```python
from build123d import *

# Parameters (mm, degrees)
F_1_4_20_TAPPED_HOLE1_D = 5.1054
SKETCH4_W               = 4.064
SKETCH4_H               = 3.0734
CHAMFER1_SIZE           = 0.127
F_8_32_TAPPED_HOLE1_D   = 3.4544
CUT_EXTRUDE1_REACH      = 182.054
SKETCH7_W               = 50.8
SKETCH7_H               = 2.565921067


with BuildPart() as part:
    # Sketch1 → Revolve1 (revolve)
    with BuildSketch(Plane.XY, mode=Mode.PRIVATE) as revolve1_sk:
        Polygon((109.7915, 0), (109.7915, 2.54), (105.7783, 2.54), (80.3783, 2.54), (80.3783, 12.7), (105.7783, 12.7), (127, 12.7), (127, 0), align=None)
    revolve(revolve1_sk.sketch.rotate(Axis((0, 0, 0), (0, 1, 0)), 90), axis=Axis((0, 0, 0), (0, 1, 0)))

    # 1/4-20 Tapped Hole1 (through all)
    with Locations(Plane(origin=(0, 12.7, 0), x_dir=(1, 0, 0), z_dir=(0, 1, 0))):
        with Locations((0, 118.745), (59.3725, 102.836186572), (102.836186572, 59.3725), (118.745, 0), (102.836186572, -59.3725), (59.3725, -102.836186572), (0, -118.745), (-59.3725, -102.836186572), (-102.836186572, -59.3725), (-118.745, 0), (-102.836186572, 59.3725), (-59.3725, 102.836186572)):
            Hole(F_1_4_20_TAPPED_HOLE1_D / 2)

    # Sketch4 → Cut-Revolve1 (revolve, cut)
    with BuildSketch(Plane.XY, mode=Mode.PRIVATE) as cut_revolve1_sk:
        with Locations((109.7788, 11.1633)):
            Rectangle(SKETCH4_W, SKETCH4_H)
    revolve(cut_revolve1_sk.sketch.rotate(Axis((0, 12.7, 0), (0, -1, 0)), 90), axis=Axis((0, 12.7, 0), (0, -1, 0)), mode=Mode.SUBTRACT)

    # Chamfer1
    chamfer1_edges = [part.edges().sort_by_distance(p)[0] for p in [
        (0, 12.7, -107.7468),
        (0, 12.7, -111.8108),
    ]]
    chamfer(chamfer1_edges, length=CHAMFER1_SIZE)

    # #8-32 Tapped Hole1 (through all)
    with Locations(Plane(origin=(0, 2.54, 0), x_dir=(-1, 0, 0), z_dir=(0, -1, 0))):
        with Locations((6.35, -85.09), (-6.35, -85.09)):
            Hole(F_8_32_TAPPED_HOLE1_D / 2)

    # Sketch7 → Cut-Extrude1 (cut, up to next)
    with BuildSketch(Plane(origin=(0, 12.7, 0), x_dir=(1, 0, 0), z_dir=(0, 1, 0)), mode=Mode.PRIVATE) as cut_extrude1_sk1:
        with Locations((0, -125.717039467)):
            Rectangle(SKETCH7_W, SKETCH7_H)
    cut_extrude1_tool1 = extrude(cut_extrude1_sk1.sketch, amount=-CUT_EXTRUDE1_REACH, mode=Mode.PRIVATE) & part.part
    add(cut_extrude1_tool1.solids().sort_by_distance((0, 12.7, 125.717039))[0], mode=Mode.SUBTRACT)


solid = part.part
```
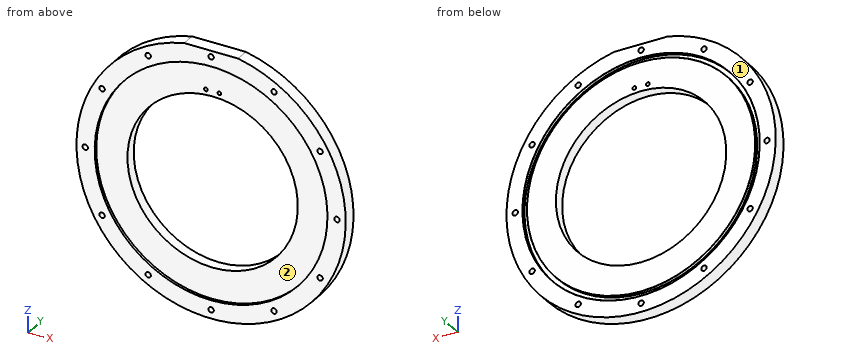
Geometry: final body of the model. Coordinates: model frame, mm. Face numbers are marked on the shaded views. Give positions to 0.01 mm unless a question says otherwise; leave off trailing zeros.
1. Section query A-A, the plane y = 7. Count the separate pieces of the cut face and the enclosed holes in it, then the cut area to 3 significant figures.
2. Pin query (flat end, axial travel): P1, Ø1.5, axis at x = -52, y = 2, coming from the +Z side; P2, Ø4, axis at x = -118.745, z = 0, coming from the -Y side; P3, Ø6, axis at y = 8.5, z = 40, coming from the -X side; P4, Ø1, axis at x = 101.5, y = 6, coming from the +Z side. Return the tip coordinate at first contact, or that it passes through.
3. Draft query along Z for the marked faces 1 and 2. Return one class per face: released by +Z, released by -Z, zero draft, split by the parting line, or undercut.
4. Line query: probe 1 along Z at (x, y) = (-6.35, 10); probe 2 along Z at (x, y) = (6.35, 9.5); probe 3 along X at (y, z) = (5.75, 85). Output: solid intervals per line, ascending.
Computed:
1. separate pieces: 1
1. enclosed holes: 15
1. area: 30,000 mm2
2. P1: stops at z = 116.2
2. P2: passes through
2. P3: stops at x = -121.49
2. P4: stops at z = 76.99
3. face 1: zero draft
3. face 2: undercut
4. probe 1: z = -126.84 to -111.63, -107.56 to -80.13, 80.13 to 83.36, 86.82 to 107.56, 111.63 to 124.43
4. probe 2: z = -126.84 to -80.13, 80.13 to 83.36, 86.82 to 124.43
4. probe 3: x = -94.36 to -8.07, -4.63 to 4.63, 8.07 to 94.36
